from build123d import *

# Parameters (mm, degrees)
BASE_FLANGE1_DEPTH = 19.05
SKETCH5_R          = 7.1501
CUT_EXTRUDE1_DEPTH = 60.846151665


# Sheet-metal steps are written as plain solids
with BuildPart() as part:
    # Sketch1 → Base-Flange1 (new, symmetric)
    with BuildSketch(Plane(origin=(0, 0, 0), x_dir=(0, 0, -1), z_dir=(1, 0, 0))):
        with BuildLine():
            Line((22.7584, 51.9684), (22.7584, 41.148))
            ThreePointArc((22.7584, 41.148), (22.609610245, 40.788789755), (22.2504, 40.64))
            Line((22.2504, 40.64), (0.254, 40.64))
            ThreePointArc((0.254, 40.64), (0.074394878, 40.565605122), (0, 40.386))
            Line((0, 40.386), (0, -40.386))
            ThreePointArc((0, -40.386), (0.074394878, -40.565605122), (0.254, -40.64))
            Line((0.254, -40.64), (22.2504, -40.64))
            ThreePointArc((22.2504, -40.64), (22.609610245, -40.788789755), (22.7584, -41.148))
            Line((22.7584, -41.148), (22.7584, -51.9684))
            Line((22.7584, -51.9684), (22.5044, -51.9684))
            Line((22.5044, -51.9684), (22.5044, -41.148))
            ThreePointArc((22.5044, -41.148), (22.430005122, -40.968394878), (22.2504, -40.894))
            Line((22.2504, -40.894), (0.254, -40.894))
            ThreePointArc((0.254, -40.894), (-0.105210245, -40.745210245), (-0.254, -40.386))
            Line((-0.254, -40.386), (-0.254, 40.386))
            ThreePointArc((-0.254, 40.386), (-0.105210245, 40.745210245), (0.254, 40.894))
            Line((0.254, 40.894), (22.2504, 40.894))
            ThreePointArc((22.2504, 40.894), (22.430005122, 40.968394878), (22.5044, 41.148))
            Line((22.5044, 41.148), (22.5044, 51.9684))
            Line((22.5044, 51.9684), (22.7584, 51.9684))
        make_face()
    extrude(amount=BASE_FLANGE1_DEPTH, both=True)

    # Sketch5 → Cut-Extrude1 (cut, through all)
    with BuildSketch(Plane.XY):
        Circle(SKETCH5_R)
    extrude(amount=CUT_EXTRUDE1_DEPTH, mode=Mode.SUBTRACT)


solid = part.part
Here's how the part is built. I have some questions about the finished solid (model axes, mm). A direction names the side the tool comes from. Coordinates: 2 decimals unless noted, no trailing zeros. Write each loop counter-clockwise with the first axis right and the second up, starting at its lowest first coordinate (ties: lowest second). Pieces come first, ordered by that corner, then holes.
Item 1: If we mould it in two halves opening along Y, with no side actions, what happens to faces 1 (the flat face through (0, -47, -22.504)), 2 (the flat face through (0, 40.64, -11)), 3 (the flat face through (0, -40.894, -11)), 4 (the flat face through (0, 40.894, -11))? For each: +Y half, -Y half, draft (parallel to the pull), parting line (faces both ways), or undercut.
Item 2: I want a section at A-A on x = 0. Write out the boundary of the cut face in (y, z).
Item 3: I want a section at C-C on z = -4.75. Write out the boundary of the cut face in (x, y), and give its area (3 significant figures).
Item 4: Will these pins go through, and if not, where does the flat tip stop? pin 1 (3 mm diameter, centred on x = -6.5, z = -3, fed in from -Y); pin 2 (8.5 mm diameter, centred on x = -1, y = 47, fed in from +Z); pin 3 (1.5 mm diameter, centred on x = 12.5, z = -2.5, fed in from +Y); pin 4 (8.5 mm diameter, centred on x = 0, y = 0, fed in from +Z).
Item 5: If I drill on line 1 (Y direction, x = -10, z = -2); line 2 (X direction, y = 0, z = 0.2); line 3 (Z direction, x = 3.5, y = -29.5), over which ranges is the centre line in solid material (lowest first)?
Item 6: I want a section at B-B on y = 0. Write out the boundary of the cut face in (x, z), and give its area (3 significant figures).
Item 7: I want a section at D-D on x = -13. Write out the boundary of the cut face in (y, z).
Item 8: On a 3-axis mill with a long thin cutter (end or side, diameter ignored), from which of +Z, -Z, +X, -X, +Y, -Y can I reach the whole of each face in a straight line? I mean faces 5 (the flat face through (0, 46, -22.504)), 6 (the flat face through (0, -40.64, -11)), 7 (the flat face through (0, -46, -22.758)). Say none if no direction works.
Findings below:
1. face 1: draft
1. face 2: undercut
1. face 3: -Y half
1. face 4: +Y half
2. outline: (-51.97, -22.76) - (-41.15, -22.76) arc R0.51 ccw to (-40.64, -22.25) - (-40.64, -0.25) arc R0.25 cw to (-40.39, 0) - (-7.15, 0) - (-7.15, 0.25) - (-40.39, 0.25) arc R0.51 ccw to (-40.89, -0.25) - (-40.89, -22.25) arc R0.25 cw to (-41.15, -22.5) - (-51.97, -22.5) - close; (7.15, 0) - (40.39, 0) arc R0.25 cw to (40.64, -0.25) - (40.64, -22.25) arc R0.51 ccw to (41.15, -22.76) - (51.97, -22.76) - (51.97, -22.5) - (41.15, -22.5) arc R0.25 cw to (40.89, -22.25) - (40.89, -0.25) arc R0.51 ccw to (40.39, 0.25) - (7.15, 0.25) - close
3. outline: (-19.05, -40.89) - (19.05, -40.89) - (19.05, -40.64) - (-19.05, -40.64) - close; (-19.05, 40.64) - (19.05, 40.64) - (19.05, 40.89) - (-19.05, 40.89) - close
3. area: 19.4 mm2
4. pin 1: stops at y = -40.89
4. pin 2: stops at z = -22.5
4. pin 3: stops at y = 40.89
4. pin 4: passes through
5. line 1: y = -40.89 to -40.64, 40.64 to 40.89
5. line 2: x = -19.05 to -7.15, 7.15 to 19.05
5. line 3: z = 0 to 0.25
6. outline: (-19.05, 0) - (-7.15, 0) - (-7.15, 0.25) - (-19.05, 0.25) - close; (7.15, 0) - (19.05, 0) - (19.05, 0.25) - (7.15, 0.25) - close
6. area: 6.05 mm2
7. outline: (-51.97, -22.76) - (-41.15, -22.76) arc R0.51 ccw to (-40.64, -22.25) - (-40.64, -0.25) arc R0.25 cw to (-40.39, 0) - (40.39, 0) arc R0.25 cw to (40.64, -0.25) - (40.64, -22.25) arc R0.51 ccw to (41.15, -22.76) - (51.97, -22.76) - (51.97, -22.5) - (41.15, -22.5) arc R0.25 cw to (40.89, -22.25) - (40.89, -0.25) arc R0.51 ccw to (40.39, 0.25) - (-40.39, 0.25) arc R0.51 ccw to (-40.89, -0.25) - (-40.89, -22.25) arc R0.25 cw to (-41.15, -22.5) - (-51.97, -22.5) - close
8. face 5: +Z, +X, -X, +Y
8. face 6: -Z, +X, -X
8. face 7: -Z, +X, -X, +Y, -Y
